Answer from the drawing. Dimensions are ordinates in mm from the lowest x, y and z of the part. Give positions to 0.01 mm unless a question says otherwise; leave off trailing zeros. Loops run counter-clockwise (first coordinate to the right, second up) from the corner with the lowest first, then second, coordinate; pieces in that order, holes last. Notation, with made-up numbers: M -22,-38.5 L 11,-38.5 A28 ccw 11,-6.5 Z; hole C 81.25,-16 d7. An arc over 180 degrees is marked long. Use a Markdown table: item, result.
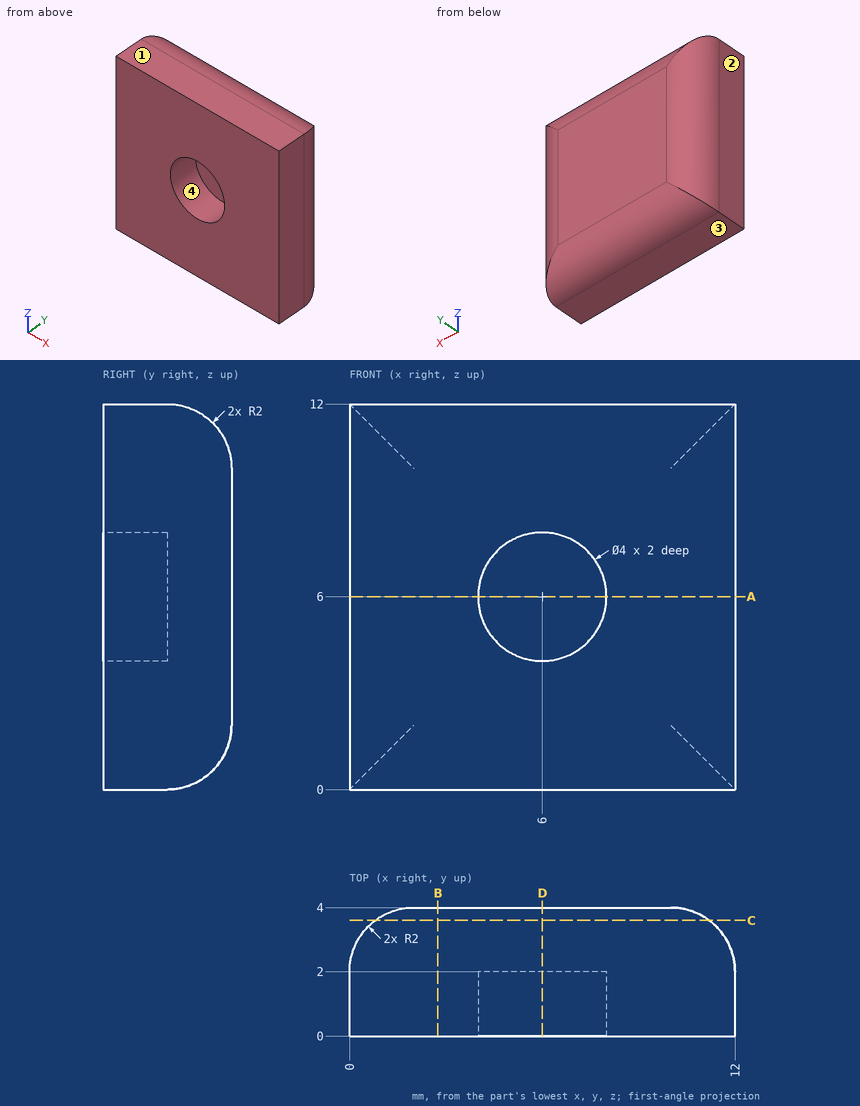
(1) The mould has two halves that part along Z. Classify the marked faces 1, 2, 3 and 4: released by +Z, released by -Z, zero draft, split by the parting line, or undercut.
Entries:
| item | result |
|---|---|
| face 1 | released by +Z |
| face 2 | zero draft |
| face 3 | released by -Z |
| face 4 | undercut |
(2) Consider probe 1 along Z at (x, y) = (6, 1.5); probe 2 along Y at (x, z) = (7.25, 7.5); probe 3 along Y at (x, z) = (1, 10). Determine where each line is inside the solid, lowest interval first. Write a range as [from, to].
Entries:
| item | result |
|---|---|
| probe 1 | z = [0, 4], [8, 12] |
| probe 2 | y = [2, 4] |
| probe 3 | y = [0, 3.73] |
(3) A cutting plane is placed at C-C (y = 3.6). Write down the section's boundary in (x, z), and give its area (3 significant figures).
Entries:
| item | result |
|---|---|
| outline | M 0.8,0.8 L 11.2,0.8 L 11.2,11.2 L 0.8,11.2 Z |
| area | 108 mm² |
(4) A cutting plane is placed at B-B (x = 2.75). Write down the section's boundary in (y, z), and give its area (3 significant figures).
Entries:
| item | result |
|---|---|
| outline | M 0,0 L 2,0 A2 ccw 4,2 L 4,10 A2 ccw 2,12 L 0,12 Z |
| area | 46.3 mm² |
(5) A cutting plane is placed at D-D (x = 6). Write down the section's boundary in (y, z), and give its area (3 significant figures).
Entries:
| item | result |
|---|---|
| outline | M 0,0 L 2,0 A2 ccw 4,2 L 4,10 A2 ccw 2,12 L 0,12 L 0,8 L 2,8 L 2,4 L 0,4 Z |
| area | 38.3 mm² |
(6) A cutting plane is placed at A-A (z = 6). Write down the section's boundary in (x, y), and give its area (3 significant figures).
Entries:
| item | result |
|---|---|
| outline | M 0,0 L 4,0 L 4,2 L 8,2 L 8,0 L 12,0 L 12,2 A2 ccw 10,4 L 2,4 A2 ccw 0,2 Z |
| area | 38.3 mm² |
(7) Given P1, Ø6, axis at x = 7.5, z = 10, coming from the -Y side; P2, Ø2, axis at x = 6, z = 6, coming from the -Y side, each flat-ended and moving along its own axis, determine where each tip first touches the part or whether it passes through.
Entries:
| item | result |
|---|---|
| P1 | stops at y = 0 |
| P2 | stops at y = 2 |
